Check sheet for the modelled part. Datum: model origin and axes. Units: mm. A direction names the side the tool comes from. Round coordinates to 2 decimals unless told otherwise and drop trailing zeros. Order: outer loops, then holes, each group sorted by start corner. A loop starts at its lowest first (then second) coordinate and runs counter-clockwise, first axis right, second up.
Q1. Mould release check, pull along X, two halves, no side actions. Record for faces 1 (the flat face through (-39.73, 2, -73)), 2 (the flat face through (-33, 0, -34)), 3 (the flat face through (-107.23, 1, -34)), 4 (the flat face through (39.77, 1, -11)): +X half, -X half, draft (parallel to the pull), parting line (faces both ways), or undercut.
Q2. Cross-section at B-B on y = 1.5. Record the cut outline in (x, z), then the cut area to 3 significant figures.
Q3. Set-up check for faces 5 (the flat face through (12, 1, -61.312)), 6 (the flat face through (-47.23, 2, -68)), 7 (the flat face through (-22, 2, -49.312)): record each of +Z, -Z, +X, -X, +Y, -Y from which the full face is reachable in a straight line by a thin tool's end or side.
Q4. Scan lines: probe 1 along X at (y, z) = (1.4, -47.5); probe 2 along Z at (x, y) = (-21, 1); probe 3 along Z at (x, y) = (-31, 0.95). Record each from-to range of solid material in increasing order.
Q5. Cross-section at A-A on z = -43.5. Record the cut outline in (x, y), then the cut area to 3 significant figures.
Q6. Cross-section at C-C on x = -10. Record the cut outline in (y, z), then the cut area to 3 significant figures.
Q7. Depth check by flat-ended pin: P1, Ø1.5, axis at x = -72, y = 1.5, coming from the -Z side; P2, Ø1.5, axis at y = 1, z = -13.5, coming from the +X side; P3, Ø0.9, axis at y = 2, z = -65.5, coming from the +X side. Enter the tip coordinate at first touch or a pass-through.
Q8. Cross-section at D-D on z = -67. Record the cut outline in (x, y).
from build123d import *

# Parameters (mm, degrees)
BOSS_EXTRUDE1_DEPTH = 3
SKETCH2_W           = 3
SKETCH2_H           = 11
CUT_EXTRUDE2_DEPTH  = 3
BOSS_EXTRUDE3_DEPTH = 3
SKETCH4_W           = 12
SKETCH4_H           = 10
CUT_EXTRUDE3_DEPTH  = 3


with BuildPart() as part:
    # Sketch1 → Boss-Extrude1 (new body)
    with BuildSketch(Plane(origin=(0, 0, 0), x_dir=(1, 0, 0), z_dir=(0, 1, 0))):
        Polygon((-104.229716691, 61.311583722), (-107.229716691, 61.311583722), (-107.229716691, 51.311583722), (-107.229716691, 6.311583722), (39.770283309, 6.311583722), (39.770283309, 16.311583722), (42.770283309, 16.311583722), (42.770283309, 61.311583722), align=None)
    extrude(amount=BOSS_EXTRUDE1_DEPTH)

    # Sketch2 → Cut-Extrude2 (cut)
    with BuildSketch(Plane(origin=(0, 3, 0), x_dir=(1, 0, 0), z_dir=(0, 1, 0))):
        with Locations((-45.729716691, 43.811583722)):
            Rectangle(SKETCH2_W, SKETCH2_H)
        with Locations((-21.729716691, 43.811583722)):
            Rectangle(SKETCH2_W, SKETCH2_H)
    extrude(amount=-CUT_EXTRUDE2_DEPTH, mode=Mode.SUBTRACT)

    # Sketch3 → Boss-Extrude3 (add)
    with BuildSketch(Plane(origin=(0, 3, 0), x_dir=(1, 0, 0), z_dir=(0, 1, 0))):
        Polygon((-47.229716691, 70.310935644), (-47.229716691, 61.311583722), (-20.229716691, 61.311583722), (-20.229716691, 70.310935644), (-20.229716691, 75.311583722), (-47.229716691, 75.311583722), align=None)
    extrude(amount=-BOSS_EXTRUDE3_DEPTH)

    # Sketch4 → Cut-Extrude3 (cut)
    with BuildSketch(Plane(origin=(0, 3, 0), x_dir=(1, 0, 0), z_dir=(0, 1, 0))):
        with Locations((-33.729716691, 75.311583722)):
            Rectangle(SKETCH4_W, SKETCH4_H)
    extrude(amount=-CUT_EXTRUDE3_DEPTH, mode=Mode.SUBTRACT)


solid = part.part
Results found:
1. face 1: undercut
1. face 2: draft
1. face 3: -X half
1. face 4: +X half
2. outline: (-107.23, -61.31) - (-47.23, -61.31) - (-47.23, -75.31) - (-39.73, -75.31) - (-39.73, -70.31) - (-27.73, -70.31) - (-27.73, -75.31) - (-20.23, -75.31) - (-20.23, -61.31) - (42.77, -61.31) - (42.77, -16.31) - (39.77, -16.31) - (39.77, -6.31) - (-107.23, -6.31) - close; hole (-47.23, -49.31) - (-44.23, -49.31) - (-44.23, -38.31) - (-47.23, -38.31) - close; hole (-23.23, -49.31) - (-20.23, -49.31) - (-20.23, -38.31) - (-23.23, -38.31) - close
2. area: 8,470 mm2
3. face 5: -Z, +X, +Y, -Y
3. face 6: -Z, -X, +Y, -Y
3. face 7: +Y, -Y
4. probe 1: x = -107.23 to -47.23, -44.23 to -23.23, -20.23 to 42.77
4. probe 2: z = -75.31 to -49.31, -38.31 to -6.31
4. probe 3: z = -70.31 to -6.31
5. outline: (-107.23, 0) - (-47.23, 0) - (-47.23, 3) - (-107.23, 3) - close; (-44.23, 0) - (-23.23, 0) - (-23.23, 3) - (-44.23, 3) - close; (-20.23, 0) - (42.77, 0) - (42.77, 3) - (-20.23, 3) - close
5. area: 432 mm2
6. outline: (0, -61.31) - (3, -61.31) - (3, -6.31) - (0, -6.31) - close
6. area: 165 mm2
7. P1: stops at z = -61.31
7. P2: stops at x = 39.77
7. P3: stops at x = -20.23
8. outline: (-47.23, 0) - (-20.23, 0) - (-20.23, 3) - (-47.23, 3) - close
